Work out the finished part from the listing and answer in its coordinate system (mm). A direction names the side the tool comes from. Coordinates: 2 decimals unless noted, no trailing zeros. Order: outer loops, then holes, each group sorted by start corner. A loop starts at its lowest first (then second) coordinate and runs counter-clockwise, first axis right, second up.
```python
from build123d import *

# Parameters (mm, degrees)
SKETCH1_W           = 38
SKETCH1_H           = 12
BOSS_EXTRUDE1_DEPTH = 1.2
SKETCH2_W           = 30
SKETCH2_H           = 11.5
BOSS_EXTRUDE2_DEPTH = 1.6
SKETCH4_W           = 24
SKETCH4_H           = 7.54
BOSS_EXTRUDE6_DEPTH = 0.1
SKETCH5_R           = 0.32
CUT_EXTRUDE1_DEPTH  = 1.2


with BuildPart() as part:
    # Sketch1 → Boss-Extrude1 (new body)
    with BuildSketch(Plane.XY):
        Rectangle(SKETCH1_W, SKETCH1_H)
    extrude(amount=BOSS_EXTRUDE1_DEPTH)

    # Sketch2 → Boss-Extrude2 (add)
    with BuildSketch(Plane.XY.offset(1.2)):
        with Locations((1, 0)):
            Rectangle(SKETCH2_W, SKETCH2_H)
    extrude(amount=BOSS_EXTRUDE2_DEPTH)

    # Sketch4 → Boss-Extrude6 (add)
    with BuildSketch(Plane.XY.offset(2.8)):
        with Locations((-0.9, 0.88)):
            Rectangle(SKETCH4_W, SKETCH4_H)
    extrude(amount=BOSS_EXTRUDE6_DEPTH)

    # Sketch5 → Cut-Extrude1 (cut)
    with BuildSketch(Plane(origin=(0, 0, 0), x_dir=(-1, 0, 0), z_dir=(0, 0, -1))):
        with Locations((17.5, 3.81)):
            Circle(SKETCH5_R)
        with Locations((17.5, 1.25)):
            Circle(SKETCH5_R)
        with Locations((17.5, -1.25)):
            Circle(SKETCH5_R)
        with Locations((17.5, -3.81)):
            Circle(SKETCH5_R)
    extrude(amount=-CUT_EXTRUDE1_DEPTH, mode=Mode.SUBTRACT)


solid = part.part
```
1. Consider probe 1 along Y at (x, z) = (-17.5, 0.7); probe 2 along Z at (x, y) = (-8.5, 4.75); probe 3 along Z at (x, y) = (-17, 1). Determine where each line is inside the solid, lowest interval first.
2. The part is cut by section B-B (x = -17.5). Determine the outline of the cut face in (y, z).
3. The part is cut by section D-D (y = 2.5). Determine the outline of the cut face in (x, z), plus the area to 3 significant figures.
4. The part is cut by section C-C (x = 3). Determine the outline of the cut face in (y, z), plus the area to 3 significant figures.
5. For faces 1 (the flat face through (1, 5.75, 2)), 2 (the flat face through (-14, 0, 2)), 3 (the flat face through (16, 0, 2)), 4 (the flat face through (1, -5.75, 2)), determine the directions among +Z, -Z, +X, -X, +Y, -Y from which every point of the face is accessible in a straight line to the end or side of a thin tool.
6. Flat-ended cylindrical pins translate along their axes: pin 1 (1.3 mm diameter, centred on y = -2, z = 2, fed in from +X); pin 2 (0.5 mm diameter, centred on x = 5, z = 1.5, fed in from +Y); pin 3 (0.5 mm diameter, centred on x = 5.5, z = 2.5, fed in from -Y). Find the tip coordinate at first contact, or state that the pin passes through.
7. The part is cut by section A-A (y = -1.25). Determine the outline of the cut face in (x, z), plus the area to 3 significant figures.
Worked out:
1. probe 1: y = -6 to -4.13, -3.49 to -1.57, -0.93 to 0.93, 1.57 to 3.49, 4.13 to 6
1. probe 2: z = 0 to 2.8
1. probe 3: z = 0 to 1.2
2. outline: (-6, 0) - (-4.13, 0) - (-4.13, 1.2) - (-6, 1.2) - close; (-3.49, 0) - (-1.57, 0) - (-1.57, 1.2) - (-3.49, 1.2) - close; (-0.93, 0) - (0.93, 0) - (0.93, 1.2) - (-0.93, 1.2) - close; (1.57, 0) - (3.49, 0) - (3.49, 1.2) - (1.57, 1.2) - close; (4.13, 0) - (6, 0) - (6, 1.2) - (4.13, 1.2) - close
3. outline: (-19, 0) - (19, 0) - (19, 1.2) - (16, 1.2) - (16, 2.8) - (11.1, 2.8) - (11.1, 2.9) - (-12.9, 2.9) - (-12.9, 2.8) - (-14, 2.8) - (-14, 1.2) - (-19, 1.2) - close
3. area: 96.0 mm2
4. outline: (-6, 0) - (6, 0) - (6, 1.2) - (5.75, 1.2) - (5.75, 2.8) - (4.65, 2.8) - (4.65, 2.9) - (-2.89, 2.9) - (-2.89, 2.8) - (-5.75, 2.8) - (-5.75, 1.2) - (-6, 1.2) - close
4. area: 33.6 mm2
5. face 1: +Z, +X, -X, +Y
5. face 2: +Z, -X, +Y, -Y
5. face 3: +Z, +X, +Y, -Y
5. face 4: +Z, +X, -X, -Y
6. pin 1: stops at x = 16
6. pin 2: stops at y = 5.75
6. pin 3: stops at y = -5.75
7. outline: (-19, 0) - (-17.82, 0) - (-17.82, 1.2) - (-19, 1.2) - close; (-17.18, 0) - (19, 0) - (19, 1.2) - (16, 1.2) - (16, 2.8) - (11.1, 2.8) - (11.1, 2.9) - (-12.9, 2.9) - (-12.9, 2.8) - (-14, 2.8) - (-14, 1.2) - (-17.18, 1.2) - close
7. area: 95.2 mm2
